```python
from build123d import *

# Parameters (mm, degrees)
F0_W     = 133.2894712687
F0_H     = 67.712135613
F1_DEPTH = 10
F2_R     = 4.99999
F3_T     = -2.5


# Not quite as in the source:
# - a fillet or chamfer is up to 0.001 mm smaller than in the source, because OpenCascade refuses the exact size


with BuildPart() as f1:
    # F0 (on Top) → F1 (new body)
    with BuildSketch(Plane.XY):
        Rectangle(F0_W, F0_H)
    extrude(amount=F1_DEPTH)

    # F2 (radius 5 in the source; OpenCascade refuses exactly that, so slightly less here)
    f2_edges = [f1.edges().sort_by_distance(p)[0] for p in [
        (66.644736, 33.856068, 5),
        (-66.644736, 33.856068, 5),
        (0, 33.856068, 0),
        (0, 33.856068, 10),
        (-66.644736, -33.856068, 5),
        (-66.644736, 0, 0),
        (-66.644736, 0, 10),
        (66.644736, -33.856068, 5),
        (0, -33.856068, 0),
        (0, -33.856068, 10),
        (66.644736, 0, 0),
        (66.644736, 0, 10),
    ]]
    fillet(f2_edges, radius=F2_R)

    # F3 (hollow: no face is removed)
    offset(amount=F3_T, mode=Mode.SUBTRACT)


solid = f1.part
```
Check sheet for the modelled part. Datum: model origin and axes. Units: mm. A direction names the side the tool comes from. Coordinates: 2 decimals unless noted, no trailing zeros. Loops run counter-clockwise (first coordinate to the right, second up) from the corner with the lowest first, then second, coordinate; pieces in that order, holes last.
1) Release check for a two-part mould opening along Y. For faces 1 (the face through (65.219, 0.404, 1.504)), 2 (the face through (-63.43, 0.4, 3.25)), 3 (the face through (0.863, -32.43, 1.504)) record: released by +Y, released by -Y, zero draft, split by the parting line, or undercut.
2) Gauge pin test, flat ends, axial feed: pin 1 (1 mm diameter, centred on y = -11, z = 2.5, fed in from +X); pin 2 (2 mm diameter, centred on x = -46.5, z = 2.5, fed in from -Y); pin 3 (3 mm diameter, centred on x = 20, z = 7, fed in from -Y). Record the tip position at first contact, or that the pin passes through.
3) Material ranges on probe 1 along Z at (x, y) = (-49.5, 5); probe 2 along Y at (x, z) = (21.5, 4.5); probe 3 along Y at (x, z) = (17, 2.75), recorded low to high.
4) Access from +Z, -Z, +X, -X, +Y, -Y to the whole of each face (thin tool, end or side, straight path). Record for faces 4 (the face through (0.86, 30.64, 6.75)), 5 (the face through (65.219, 0.404, 8.496)).
5) Sectioned sample at C-C (z = 1.25). Record the boundary of the cut face in (x, y).
Check sheet entries:
1. face 1: zero draft
1. face 2: undercut
1. face 3: released by -Y
2. pin 1: stops at x = 66.23
2. pin 2: stops at y = -33.63
2. pin 3: stops at y = -33.83
3. probe 1: z = 0 to 2.5, 7.5 to 10
3. probe 2: y = -33.83 to -31.31, 31.31 to 33.83
3. probe 3: y = -33.32 to -29.95, 29.95 to 33.32
4. face 4: none
4. face 5: +Z, +X, +Y, -Y
5. outline: (-64.95, -28.86) arc R3.31 ccw to (-61.64, -32.16) - (61.64, -32.16) arc R3.31 ccw to (64.95, -28.86) - (64.95, 28.86) arc R3.31 ccw to (61.64, 32.16) - (-61.64, 32.16) arc R3.31 ccw to (-64.95, 28.86) - close
